Autodesk Inventor part; units mm, degrees
ref_plane "YZ Plane" through (0, 0, 0) normal (1, 0, 0) x (0, 1, 0)
ref_plane "XZ Plane" through (0, 0, 0) normal (0, 1, 0) x (-1, 0, 0)
ref_plane "XY Plane" through (0, 0, 0) normal (0, 0, 1) x (1, 0, 0)
sketch "Sketch1" plane through (0, 0, 0) normal (0, 1, 0) x (-1, 0, 0)
  arc A0 (-1.5117, -19.1905) -> (1.5117, -19.1905) centre (0, -20.5) ccw
  circle A1 centre (0, 20.5) radius 1
  circle A2 centre (0, -20.5) radius 1
  arc A3 (-1.5117, 19.1905) -> (-19.1905, 1.5118) centre (0, 0) ccw
  arc A4 (-19.1905, 1.5118) -> (-19.1905, -1.5118) centre (-20.4999, 0) ccw
  arc A5 (-19.1905, -1.5118) -> (-1.5117, -19.1905) centre (0, 0) ccw
  arc A6 (-1.5117, -19.1905) -> (1.5117, -19.1905) centre (0, -20.5) ccw
  arc A7 (1.5117, -19.1905) -> (19.1909, -1.5076) centre (0, 0) ccw
  arc A8 (19.1909, -1.5076) -> (19.1909, 1.5076) centre (20.505, 0) ccw
  arc A9 (19.1909, 1.5076) -> (1.5117, 19.1905) centre (0, 0) ccw
  arc A10 (1.5117, 19.1905) -> (-1.5117, 19.1905) centre (0, 20.5) ccw
  circle A11 centre (-20.4999, 0) radius 1
  arc A12 (-18.5, -0.0197) -> (-18.5, 0.0197) centre (-20.4999, 0) ccw
  circle A13 centre (20.505, 0) radius 1
extrude "Extrusion1" add sketch "Sketch1" along normal blind 1.5
properties part number "tapaRGB-anillo"
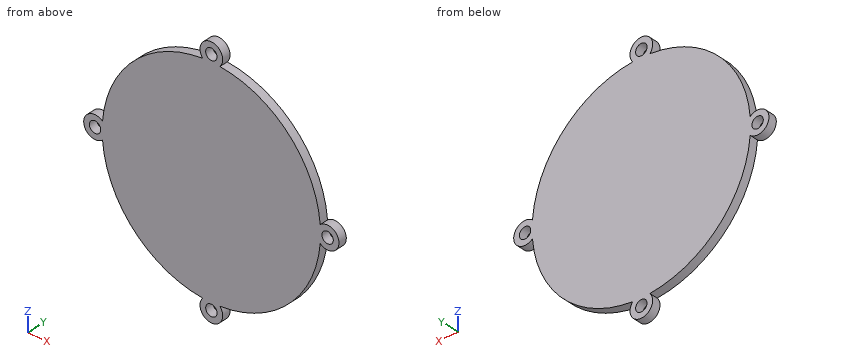
Design review of the part built by this model. Coordinates are the model's own, in mm. Round coordinates to 2 decimals unless told otherwise and drop trailing zeros. Write each loop counter-clockwise with the first axis right and the second up, starting at its lowest first coordinate (ties: lowest second). Pieces come first, ordered by that corner, then holes. Notation, with made-up numbers: (61, 15.5) -> (99, 15.5) arc R20 ccw to (99, 40.5) -> close; hole circle Ø7 at (77, 73.5). An arc over 180 degrees is marked (long way). One line per item, written item: value. Start each with the question number.
Q1. Add section C-C (z = -20.5). Give the boundary of the cut face in (x, y), then the cut area to 3 significant figures.
Q2. Add section A-A (x = 0). Give the boundary of the cut face in (y, z), then the cut area to 3 significant figures.
Q3. Add section B-B (y = 0.65). Give the boundary of the cut face in (x, z) (1 decimal).
Q4. Add section D-D (z = 15.5). Give the boundary of the cut face in (x, y).
Q5. Insertion check: P1, Ø3, axis at x = 0, z = -20.5, coming from the +Y side; P2, Ø1.6, axis at x = 20.5, z = 0, coming from the -Y side. Each pin has a flat end and moves straight along its axis. Give the tip position at first contact, or say it passes through.
Q6. To check wall thickness, follow probe 1 along Z at (x, y) = (0, 0.6); probe 2 along Z at (x, y) = (-4.5, 1.45); probe 3 along X at (y, z) = (0.9, 6). State the ranges of each line that lie inside material, in increasing order.
Response:
1. outline: (-2, 0) -> (-1, 0) -> (-1, 1.5) -> (-2, 1.5) -> close; (1, 0) -> (2, 0) -> (2, 1.5) -> (1, 1.5) -> close
1. area: 3.00 mm^2
2. outline: (0, -22.5) -> (1.5, -22.5) -> (1.5, -21.5) -> (0, -21.5) -> close; (0, -19.5) -> (1.5, -19.5) -> (1.5, 19.5) -> (0, 19.5) -> close; (0, 21.5) -> (1.5, 21.5) -> (1.5, 22.5) -> (0, 22.5) -> close
2. area: 61.5 mm^2
3. outline: (-19.2, -1.5) arc R19.3 ccw to (-1.5, -19.2) arc R2 ccw (long way) to (1.5, -19.2) arc R19.2 ccw to (19.2, -1.5) arc R2 ccw (long way) to (19.2, 1.5) arc R19.2 ccw to (1.5, 19.2) arc R2 ccw (long way) to (-1.5, 19.2) arc R19.2 ccw to (-19.2, 1.5) arc R2 ccw (long way) to start; hole circle Ø2 at (-20.5, 0); hole circle Ø2 at (0, -20.5); hole circle Ø2 at (0, 20.5); hole circle Ø2 at (20.5, 0)
4. outline: (-11.42, 0) -> (11.42, 0) -> (11.42, 1.5) -> (-11.42, 1.5) -> close
5. P1: stops at y = 1.5
5. P2: passes through
6. probe 1: z = -22.5 to -21.5, -19.5 to 19.5, 21.5 to 22.5
6. probe 2: z = -18.72 to 18.72
6. probe 3: x = -18.29 to 18.29
